```python
from build123d import *

# Parameters (mm, degrees)
SKETCH1_R           = 7
SKETCH1_R_2         = 10
SKETCH1_R_3         = 1.5
SKETCH1_R_4         = 1.75
BOSS_EXTRUDE1_DEPTH = 5


with BuildPart() as part:
    # Sketch1 → Boss-Extrude1 (new body)
    with BuildSketch(Plane.XY):
        with BuildLine():
            Line((-71.071428571, 14.961685761), (-1.428571429, 19.948914348))
            ThreePointArc((-1.428571429, 19.948914348), (-0.686118829, 19.988227559), (0.057281956, 19.999917969))
            Line((0.057281956, 19.999917969), (8.242983117, 34.177968276))
            ThreePointArc((8.242983117, 34.177968276), (9.441459784, 35.47447303), (11.081346872, 36.128721638))
            Line((11.081346872, 36.128721638), (24.727055657, 38.289989587))
            ThreePointArc((24.727055657, 38.289989587), (29.30354688, 34.964974085), (25.978531377, 30.388482862))
            Line((25.978531377, 30.388482862), (16.101647971, 28.824138212))
            ThreePointArc((16.101647971, 28.824138212), (14.461760884, 28.169889604), (13.263284216, 26.873384849))
            Line((13.263284216, 26.873384849), (8.263284216, 18.213130812))
            ThreePointArc((8.263284216, 18.213130812), (19.384626574, -4.923032864), (-1.428571429, -19.948914348))
            Line((-1.428571429, -19.948914348), (-71.071428571, -14.961685761))
            ThreePointArc((-71.071428571, -14.961685761), (-85, 0), (-71.071428571, 14.961685761))
        make_face()
        with Locations((-70, 0)):
            Circle(SKETCH1_R, mode=Mode.SUBTRACT)
        Circle(SKETCH1_R_2, mode=Mode.SUBTRACT)
        with Locations((-12.903778516, 7.45)):
            Circle(SKETCH1_R_3, mode=Mode.SUBTRACT)
        with Locations((0, -14.9)):
            Circle(SKETCH1_R_3, mode=Mode.SUBTRACT)
        with Locations((-27.262321561, 14.088677781)):
            Circle(SKETCH1_R_4, mode=Mode.SUBTRACT)
        with Locations((-27.262321561, -14.088677781)):
            Circle(SKETCH1_R_4, mode=Mode.SUBTRACT)
        with Locations((12.903778516, 7.45)):
            Circle(SKETCH1_R_3, mode=Mode.SUBTRACT)
        with Locations((25.352793517, 34.339236225)):
            Circle(SKETCH1_R_3, mode=Mode.SUBTRACT)
    extrude(amount=BOSS_EXTRUDE1_DEPTH)


with BuildPart() as part_1:
    # Body-Move/Copy1: moved
    add(part.part.moved(Location((0, 0, -5))))


solid = part_1.part
```
For this review, take the finished solid that the model builds, in its own axes (mm). A direction names the side the tool comes from. Give positions to 0.01 mm unless a question says otherwise; leave off trailing zeros. Write each loop counter-clockwise with the first axis right and the second up, starting at its lowest first coordinate (ties: lowest second). Pieces come first, ordered by that corner, then holes.
Item 1: Insertion check: P1, Ø1.8, axis at x = 25.35, y = 34.34, coming from the +Z side; P2, Ø1.5, axis at x = -31, z = -3, coming from the +Y side; P3, Ø3, axis at x = -19, z = -2, coming from the +Y side. Each pin has a flat end and moves straight along its axis. Give the tip position at first contact, or say it passes through.
Item 2: Take a section at C-C (z = -1.2). Give the number of separate pieces and of enclosed holes in the cut face, and give its area (3 significant figures).
Item 3: Machinability: for faces 4 (the face through (-27, 3, -5)), 5 (the face through (14.48, 28.18, -2.54)), which of the approach directions +Z, -Z, +X, -X, +Y, -Y give a long, thin tool a straight path to every point of the face, cutting with its end or side? Answer none if there is none.
Item 4: Take a section at A-A (y = -2). Give the boundary of the cut face in (x, z).
Item 5: Take a section at B-B (x = -8). Give the boundary of the cut face in (y, z), and give its area (3 significant figures).
Item 6: The part is to be moulded in two halves that separate along Y. For faces 1 (the face through (17.809, 37.194, -2.535)), 2 (the face through (-25.646, 13.418, -2.535)), 3 (the face through (-85, 0, -3)), say which applies: +Y half, -Y half, draft (parallel to the pull), parting line (faces both ways), or undercut.
Item 7: Wall thickness on probe 1 along X at (y, z) = (0.5, -3.75); probe 2 along Y at (x, z) = (0, -3.4); probe 3 along X at (y, z) = (2, -3.15): over which ranges is each line inside the solid? List them lowest first.
Item 8: Take a section at D-D (x = -70). Give the boundary of the cut face in (y, z).
Established:
1. P1: passes through
1. P2: stops at y = 17.88
1. P3: stops at y = 18.8
2. separate pieces: 1
2. enclosed holes: 8
2. area: 3,180 mm2
3. face 4: -Z, +X, -X, +Y, -Y
3. face 5: +Z, -Z, +X
4. outline: (-84.87, -5) - (-76.71, -5) - (-76.71, 0) - (-84.87, 0) - close; (-63.29, -5) - (-9.8, -5) - (-9.8, 0) - (-63.29, 0) - close; (9.8, -5) - (19.9, -5) - (19.9, 0) - (9.8, 0) - close
5. outline: (-19.48, -5) - (-6, -5) - (-6, 0) - (-19.48, 0) - close; (6, -5) - (19.48, -5) - (19.48, 0) - (6, 0) - close
5. area: 135 mm2
6. face 1: +Y half
6. face 2: undercut
6. face 3: parting line
7. probe 1: x = -84.99 to -76.98, -63.02 to -9.99, 9.99 to 19.99
7. probe 2: y = -20 to -16.4, -13.4 to -10, 10 to 20
7. probe 3: x = -84.87 to -76.71, -63.29 to -9.8, 9.8 to 19.9
8. outline: (-15.04, -5) - (-7, -5) - (-7, 0) - (-15.04, 0) - close; (7, -5) - (15.04, -5) - (15.04, 0) - (7, 0) - close
